Verification items for the finished model (mm, model axes). A direction names the side the tool comes from. Give positions to 0.01 mm unless a question says otherwise; leave off trailing zeros. Loops run counter-clockwise (first coordinate to the right, second up) from the corner with the lowest first, then second, coordinate; pieces in that order, holes last. Notation, with made-up numbers: (26, -14) -> (68, -14) arc R24 cw to (68, 18) -> close; hole circle Ø8 at (-12, 79.5). An arc over 180 degrees is marked (long way). Answer in a Markdown table with one row per item. Add a question column.
Q1. Section check B-B on z = 1.65. Enter the section's corners in (x, y), and give its area (3 significant figures).
Q2. Set-up check for faces 1 (the face through (0.262, 11.897, 1.479)), 2 (the face through (4.052, -0.086, -1.479)): record each of +Z, -Z, +X, -X, +Y, -Y from which the full face is reachable in a straight line by a thin tool's end or side.
Q3. Section check A-A on y = -6. Enter the section's corners in (x, z).
Q4. Section check D-D on x = 0. Enter the section's corners in (y, z), and give its area (3 significant figures).
Q5. Material ranges on probe 1 along X at (y, z) = (-18, 1.6); probe 2 along Z at (x, y) = (-8, -20); probe 3 along Y at (x, z) = (-6.9, 1.6), recorded low to high.
Q6. Section check C-C on x = 6.9. Enter the section's corners in (y, z) (3 decimals).
Q7. Release check for a two-part mould opening along Y. For faces 3 (the face through (-0.423, 7.904, -1.479)), 4 (the face through (-7.948, -0.086, -1.479)), 5 (the face through (0, -5, 3)), 6 (the face through (6, -19.73, 1.47)) record: pulls with the +Y half, pulls with the -Y half, needs draft (parallel to the pull), parting line crosses it, or undercut.
Q8. Gauge pin test, flat ends, axial feed: P1, Ø1, axis at x = 9.5, z = -2.5, coming from the -Y side; P2, Ø6, axis at x = 6.9, y = -18, coming from the -Z side. Record the tip position at first contact, or that the pin passes through.
```python
from build123d import *

# Parameters (mm, degrees)
BOSS_EXTRUDE1_DEPTH              = 3
SKETCH2_R                        = 1.95
BOSS_EXTRUDE2_DEPTH              = 3
M3_5_CLEARANCE_HOLE1_D           = 3.9
M3_5_CLEARANCE_HOLE1_CSINK_D     = 3.95
M3_5_CLEARANCE_HOLE1_CSINK_ANGLE = 90


with BuildPart() as part:
    # Sketch1 → Boss-Extrude1 (new body)
    with BuildSketch(Plane.XY):
        with BuildLine():
            Line((-11.9, 0), (-11.9, -22))
            Line((-11.9, -22), (11.9, -22))
            Line((11.9, -22), (11.9, 0))
            ThreePointArc((11.9, 0), (0, 11.9), (-11.9, 0))
        make_face()
    extrude(amount=BOSS_EXTRUDE1_DEPTH)

    # Sketch2 → Boss-Extrude2 (add)
    with BuildSketch(Plane(origin=(0, 0, 0), x_dir=(-1, 0, 0), z_dir=(0, 0, -1))):
        with Locations(Location((0, 6, 0), (0, 0, 180))):
            Circle(SKETCH2_R)
        with Locations(Location((6, 0, 0), (0, 0, 180))):
            Circle(SKETCH2_R)
        with Locations(Location((0, -6, 0), (0, 0, 180))):
            Circle(SKETCH2_R)
        with Locations(Location((-6, 0, 0), (0, 0, 180))):
            Circle(SKETCH2_R)
    extrude(amount=BOSS_EXTRUDE2_DEPTH)

    # M3.5 Clearance Hole1 (through all)
    with Locations(Plane.XY.offset(3)):
        with Locations((6.9, -18), (-6.9, -18)):
            CounterSinkHole(M3_5_CLEARANCE_HOLE1_D / 2, M3_5_CLEARANCE_HOLE1_CSINK_D / 2, counter_sink_angle=M3_5_CLEARANCE_HOLE1_CSINK_ANGLE)


solid = part.part
```
Taken from the geometry:
| question | item | result |
|---|---|---|
| 1 | outline | (-11.9, -22) -> (11.9, -22) -> (11.9, 0) arc R11.9 ccw to (-11.9, 0) -> close; hole circle Ø3.9 at (-6.9, -18); hole circle Ø3.9 at (6.9, -18) |
| 1 | area | 722 mm² |
| 2 | face 1 | +Z, -Z, +Y |
| 2 | face 2 | -Z |
| 3 | outline | (-11.9, 0) -> (-1.95, 0) -> (-1.95, -3) -> (1.95, -3) -> (1.95, 0) -> (11.9, 0) -> (11.9, 3) -> (-11.9, 3) -> close |
| 4 | outline | (-22, 0) -> (-7.95, 0) -> (-7.95, -3) -> (-4.05, -3) -> (-4.05, 0) -> (4.05, 0) -> (4.05, -3) -> (7.95, -3) -> (7.95, 0) -> (11.9, 0) -> (11.9, 3) -> (-22, 3) -> close |
| 4 | area | 125 mm² |
| 5 | probe 1 | x = -11.9 to -8.85, -4.95 to 4.95, 8.85 to 11.9 |
| 5 | probe 2 | z = 0 to 3 |
| 5 | probe 3 | y = -22 to -19.95, -16.05 to 9.7 |
| 6 | outline | (-22, 0) -> (-19.95, 0) -> (-19.95, 2.975) -> (-19.975, 3) -> (-22, 3) -> close; (-16.05, 0) -> (-1.73, 0) -> (-1.73, -3) -> (1.73, -3) -> (1.73, 0) -> (9.695, 0) -> (9.695, 3) -> (-16.025, 3) -> (-16.05, 2.975) -> close |
| 7 | face 3 | undercut |
| 7 | face 4 | parting line crosses it |
| 7 | face 5 | needs draft |
| 7 | face 6 | undercut |
| 8 | P1 | passes through |
| 8 | P2 | stops at z = 0 |
